For this review, take the finished solid that the model builds, in its own axes (mm). Face numbers are marked on the shaded views. Give positions to 0.01 mm unless a question says otherwise; leave off trailing zeros. Loops run counter-clockwise (first coordinate to the right, second up) from the corner with the lowest first, then second, coordinate; pieces in that order, holes last. Notation, with made-up numbers: (53.25, -31) - (104.25, -31) arc R32 ccw to (104.25, 7) - close; hole circle Ø5 at (-12.75, 71). An arc over 180 degrees is marked (long way). Use CSV: the item, a comma, the result in double quotes. Start each with the question number.
1. Take a section at B-B on y = 0. Give the boundary of the cut face in (x, z) (3 decimals).
2. Take a section at C-C on z = 50. Give the boundary of the cut face in (x, y) (3 decimals), plus the area to 3 significant figures.
3. For pin 1 (6 mm diameter, centred on x = -12.5, z = 45.5, fed in from +Y); pin 2 (4.5 mm diameter, centred on y = 0, z = 50, fed in from -X); pin 3 (5 mm diameter, centred on y = -12.5, z = 25.5, fed in from +X); pin 4 (6 mm diameter, centred on y = -11, z = 39, fed in from -X), all flat-tipped, find the tip position at first contact; note any pin that passes through.
4. Take a section at D-D on z = 38. Give the boundary of the cut face in (x, y) (3 decimals).
5. Mouldability with a two-part tool opening along Y and no side actions: class the marked faces 1 and 2 as pulls with the +Y half, pulls with the -Y half, needs draft (parallel to the pull), parting line crosses it, or undercut.
6. Wall thickness on line 1 (X direction, y = 0, z = 41.5) (3 decimals); line 2 (Z direction, x = 14.75, y = 0): over which ranges is each line inside the solid? List them lowest first.
7. Take a section at A-A on x = 0. Give the boundary of the cut face in (y, z) (3 decimals).
```python
from build123d import *

# Parameters (mm, degrees)
F0_R     = 15.875
F0_R_2   = 13.875
F1_DEPTH = 62
F2_R     = 2.5
F3_DEPTH = 25


with BuildPart() as f1:
    # F0 (on Top) → F1 (new body)
    with BuildSketch(Plane.XY):
        Circle(F0_R)
        Circle(F0_R_2, mode=Mode.SUBTRACT)
    extrude(amount=F1_DEPTH)

    # F2 (on Right) → F3 (cut, symmetric)
    with BuildSketch(Plane.YZ):
        with Locations((0, 50)):
            Circle(F2_R)
        with Locations((0, 25)):
            Circle(F2_R)
    extrude(amount=F3_DEPTH, both=True, mode=Mode.SUBTRACT)


solid = f1.part
```
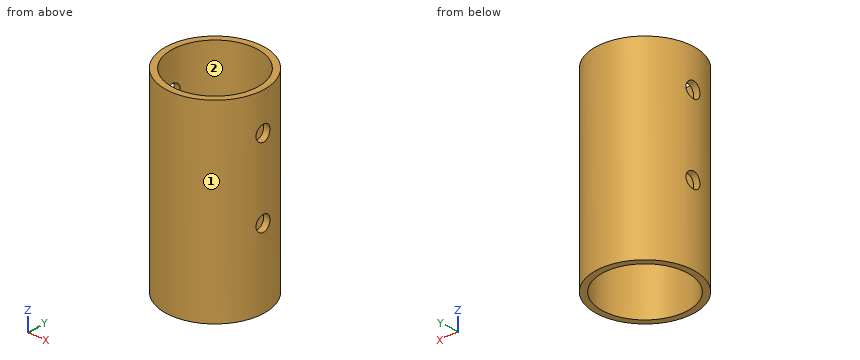
Check result:
1,outline,"(-15.875, 0) - (-13.875, 0) - (-13.875, 22.5) - (-15.875, 22.5) - close; (-15.875, 27.5) - (-13.875, 27.5) - (-13.875, 47.5) - (-15.875, 47.5) - close; (-15.875, 52.5) - (-13.875, 52.5) - (-13.875, 62) - (-15.875, 62) - close; (13.875, 0) - (15.875, 0) - (15.875, 22.5) - (13.875, 22.5) - close; (13.875, 27.5) - (15.875, 27.5) - (15.875, 47.5) - (13.875, 47.5) - close; (13.875, 52.5) - (15.875, 52.5) - (15.875, 62) - (13.875, 62) - close"
2,outline,"(-15.677, -2.5) arc R15.875 ccw to (15.677, -2.5) - (13.648, -2.5) arc R13.875 cw to (-13.648, -2.5) - close; (-15.677, 2.5) - (-13.648, 2.5) arc R13.875 cw to (13.648, 2.5) - (15.677, 2.5) arc R15.875 ccw to start"
2,area,"167 mm²"
3,pin 1,"stops at y = 12.72"
3,pin 2,"passes through"
3,pin 3,"stops at x = 12.33"
3,pin 4,"stops at x = -13.71"
4,outline,"circle Ø31.75 at (0, 0); hole circle Ø27.75 at (0, 0)"
5,face 1,"parting line crosses it"
5,face 2,"undercut"
6,line 1,"x = -15.875 to -13.875, 13.875 to 15.875"
6,line 2,"z = 0 to 22.5, 27.5 to 47.5, 52.5 to 62"
7,outline,"(-15.875, 0) - (-13.875, 0) - (-13.875, 62) - (-15.875, 62) - close; (13.875, 0) - (15.875, 0) - (15.875, 62) - (13.875, 62) - close"
